Verification items for the finished model (mm, model axes). Give positions to 0.01 mm unless a question says otherwise; leave off trailing zeros. Order: outer loops, then holes, each group sorted by start corner. A loop starts at its lowest first (then second) coordinate and runs counter-clockwise, first axis right, second up. Notation, with made-up numbers: (43, 44.5) -> (78, 44.5) arc R31 ccw to (78, 79.5) -> close; hole circle Ø8 at (39, 40.25). An arc over 180 degrees is marked (long way). Return JSON: item names as keys, results as strings. Group by question number.
(1) Cross-section at D-D on z = 2. State how many separate pieces and enclosed holes the cut face has, then the cut area to 3 significant figures.
(2) Release check for a two-part mould opening along Y. For faces 1 (the face through (25.21, -0.01, 5.07)), 2 (the face through (22, -4, 0)), 3 (the face through (1.736, -7.671, 4.93)) record: pulls with the +Y half, pulls with the -Y half, needs draft (parallel to the pull), parting line crosses it, or undercut.
(3) Thickness scan on line 1 along Y through (x, z) = (23.5, 3); line 2 along X through (y, z) = (-0.5, 1.5); line 3 along X through (y, z) = (2.5, 6.75). Record the ranges inside material, lowest first.
(4) Cross-section at C-C on x = 17.82. Enter the section's corners in (y, z).
(5) Depth check by flat-ended pin: pin 1 Ø5 at (x, y) = (15.41, -10.04) entering from -Z; pin 2 Ø6 at (x, z) = (4.5, 2) entering from +Y. Enter the tip coordinate at first touch or a pass-through.
(6) Cross-section at B-B on y = 15. Enter the section's corners in (x, z).
(7) Cross-section at A-A on x = 7. Enter the section's corners in (y, z).
from build123d import *

# Parameters (mm, degrees)
CYLINDER_R        = 3.2
CYLINDER_DEPTH    = 10
ARRAY_COUNT       = 7
CYLINDER001_R     = 17.82
CYLINDER001_DEPTH = 10
SKETCH001_R       = 4.5
SKETCH001_R_2     = 3
POCKET_DEPTH      = 10.001


with BuildPart() as obj1:
    # Cylinder → Cylinder (new body)
    with BuildSketch(Plane.XY):
        Circle(CYLINDER_R)
    extrude(amount=CYLINDER_DEPTH)

    # Array: obj1 ×7 about axis
    array_axis = Axis((17.82, 0, 0), (0, 0, 1))


with BuildPart() as obj1_1:
    add(obj1.part)
    for i in range(1, ARRAY_COUNT):
        add(obj1.part.rotate(array_axis, i * 360 / ARRAY_COUNT))


with BuildPart() as obj2:
    # Cylinder001 → Cylinder001 (new body)
    with BuildSketch(Plane(origin=(17.82, 0, 0), x_dir=(1, 0, 0), z_dir=(0, 0, 1))):
        Circle(CYLINDER001_R)
    extrude(amount=CYLINDER001_DEPTH)

    # Cut: cut obj1
    add(obj1_1.part, mode=Mode.SUBTRACT)

    # Sketch001 → Pocket (cut, through all)
    with BuildSketch(Plane.XY.offset(10)):
        with Locations((17.82, -0.034345)):
            Circle(SKETCH001_R)
        with Locations((15.621058, 9.35508)):
            Circle(SKETCH001_R_2)
        with Locations((23.669142, 7.910553)):
            Circle(SKETCH001_R_2)
        with Locations((28.209085, -0.137526)):
            Circle(SKETCH001_R_2)
        with Locations((23.875502, -8.185606)):
            Circle(SKETCH001_R_2)
        with Locations((15.414699, -10.042854)):
            Circle(SKETCH001_R_2)
        with Locations((8.192065, -4.677468)):
            Circle(SKETCH001_R_2)
        with Locations((8.707965, 4.196056)):
            Circle(SKETCH001_R_2)
    extrude(amount=-POCKET_DEPTH, mode=Mode.SUBTRACT)


solid = obj2.part
Verdict:
{
 "1": {"separate pieces": "1", "enclosed holes": "8", "area": "628 mm²"},
 "2": {"face 1": "undercut", "face 2": "needs draft", "face 3": "pulls with the -Y half"},
 "3": {"line 1": "-14.67 to -11.16, -5.21 to 4.92, 10.91 to 14.67", "line 2": "3.16 to 13.34, 22.3 to 25.23, 31.19 to 35.63", "line 3": "2 to 6.23, 11.18 to 14.1, 21.54 to 26.78, 29.64 to 35.46"},
 "4": {"outline": "(-17.82, 0) -> (-11.84, 0) -> (-11.84, 10) -> (-17.82, 10) -> close; (-8.25, 0) -> (-4.53, 0) -> (-4.53, 10) -> (-8.25, 10) -> close; (4.47, 0) -> (7.31, 0) -> (7.31, 10) -> (4.47, 10) -> close; (11.4, 0) -> (17.82, 0) -> (17.82, 10) -> (11.4, 10) -> close"},
 "5": {"pin 1": "through", "pin 2": "y = 11.72"},
 "6": {"outline": "(9.73, 0) -> (19.64, 0) -> (19.64, 10) -> (9.73, 10) -> close; (23.93, 0) -> (27.44, 0) -> (27.44, 10) -> (23.93, 10) -> close"},
 "7": {"outline": "(-10.75, 0) -> (-7.43, 0) -> (-7.43, 10) -> (-10.75, 10) -> close; (-1.92, 0) -> (1.73, 0) -> (1.73, 10) -> (-1.92, 10) -> close; (6.66, 0) -> (10.75, 0) -> (10.75, 10) -> (6.66, 10) -> close"}
}
